Part model, mm, in its own coordinate system. Round coordinates to 2 decimals unless told otherwise and drop trailing zeros. Write each loop counter-clockwise with the first axis right and the second up, starting at its lowest first coordinate (ties: lowest second). Pieces come first, ordered by that corner, then holes. Notation, with made-up numbers: (29.25, -14.5) -> (52.25, -14.5) arc R26 ccw to (52.25, 23.5) -> close; hole circle Ø9 at (37.5, -35.75). An arc over 180 degrees is marked (long way). Return JSON: item names as keys, results as strings. Group by question number.
(1) Saw through at B-B (y = 1.3). List the corners of the cut face in (x, z), plus the area to 3 significant figures.
(2) Drill centre lines: L1, parallel to X at y = 1, z = 0; L2, parallel to X at y = 0.6, z = -16.5; L3, parallel to Z at x = 7.5, y = 0.7. Where is each one in solid material? Low to high. Write a range as from..to.
(3) Saw through at A-A (z = 0). List the corners of the cut face in (x, y).
(4) Mould opens along Z. For faces 1 (the flat face through (0, 1, -20)), 2 (the flat face through (0, 1, 20)), 3 (the flat face through (0, 2, 0)), 4 (the cylindrical face through (-16.78, 0.99, 15.24)) say: +Z half, -Z half, draft (parallel to the pull), parting line (faces both ways), or undercut.
from build123d import *

# Parameters (mm, degrees)
SKETCH1_W               = 40.64
SKETCH1_H               = 39.9999962
BOSS_EXTRUDE1_DEPTH     = 1.999996
CUT_EXTRUDE1_DEPTH      = 29.5815029
CUT_EXTRUDE1_DEPTH_BACK = 29.5815029
SKETCH2_R               = 1.877518959
SKETCH2_R_2             = 1.749160226


with BuildPart() as part:
    # Sketch1 → Boss-Extrude1 (new body)
    with BuildSketch(Plane(origin=(0, 0, 0), x_dir=(1, 0, 0), z_dir=(0, 1, 0))):
        Rectangle(SKETCH1_W, SKETCH1_H)
    extrude(amount=BOSS_EXTRUDE1_DEPTH)

    # Sketch2 → Cut-Extrude1 (cut, two sides: drawn at the far end of the back side and taken through both)
    with BuildSketch(Plane(origin=(0, 1.999996, 0), x_dir=(1, 0, 0), z_dir=(0, 1, 0)).offset(-CUT_EXTRUDE1_DEPTH_BACK)):
        with Locations((-18.654170648, 15.167488224)):
            Circle(SKETCH2_R)
        with Locations((-18.654170648, -15.167488224)):
            Circle(SKETCH2_R)
        with Locations((18.654170648, -15.167488224)):
            Circle(SKETCH2_R)
        with Locations((18.654170648, 15.167488224)):
            Circle(SKETCH2_R)
        with Locations(Location((-7.497989174, 0, 0), (0, 0, 270))):
            Circle(SKETCH2_R_2)
        with Locations(Location((7.497989174, 0, 0), (0, 0, 90))):
            Circle(SKETCH2_R_2)
    extrude(amount=CUT_EXTRUDE1_DEPTH + CUT_EXTRUDE1_DEPTH_BACK, mode=Mode.SUBTRACT)


solid = part.part
Computed values:
{
 "1": {"outline": "(-20.32, -20) -> (20.32, -20) -> (20.32, -16.03) arc R1.88 cw (long way) to (20.32, -14.3) -> (20.32, 14.3) arc R1.88 cw (long way) to (20.32, 16.03) -> (20.32, 20) -> (-20.32, 20) -> (-20.32, 16.03) arc R1.88 cw (long way) to (-20.32, 14.3) -> (-20.32, -14.3) arc R1.88 cw (long way) to (-20.32, -16.03) -> close; hole circle Ø3.5 at (-7.5, 0); hole circle Ø3.5 at (7.5, 0)", "area": "1,560 mm2"},
 "2": {"L1": "-20.32..-9.25, -5.75..5.75, 9.25..20.32", "L2": "-20.32..-19.98, -17.33..17.33, 19.98..20.32", "L3": "-20..-1.75, 1.75..20"},
 "3": {"outline": "(-20.32, 0) -> (-9.25, 0) -> (-9.25, 2) -> (-20.32, 2) -> close; (-5.75, 0) -> (5.75, 0) -> (5.75, 2) -> (-5.75, 2) -> close; (9.25, 0) -> (20.32, 0) -> (20.32, 2) -> (9.25, 2) -> close"},
 "4": {"face 1": "-Z half", "face 2": "+Z half", "face 3": "draft", "face 4": "undercut"}
}
